Geometry check sheet. Reference: the model listing, model coordinates, mm. A direction names the side the tool comes from. Coordinates: 2 decimals unless noted, no trailing zeros. Loops run counter-clockwise (first coordinate to the right, second up) from the corner with the lowest first, then second, coordinate; pieces in that order, holes last.
from build123d import *

# Parameters (mm, degrees)
SKETCH1_W            = 299.7
SKETCH1_H            = 76.075
BOSS_EXTRUDE1_DEPTH  = 3.175
CUT_EXTRUDE4_DEPTH   = 155.634907221
SKETCH3_R            = 6.5
CUT_EXTRUDE5_DEPTH   = 155.634907221
M4_CLEARANCE_HOLE1_D = 4.5
SKETCH12_W           = 144
SKETCH12_H           = 3.175
BOSS_EXTRUDE2_DEPTH  = 6.35
SKETCH13_R           = 14
CUT_EXTRUDE6_DEPTH   = 157.318115653


with BuildPart() as part:
    # Sketch1 → Boss-Extrude1 (new body)
    with BuildSketch(Plane.XY):
        Rectangle(SKETCH1_W, SKETCH1_H)
    extrude(amount=BOSS_EXTRUDE1_DEPTH)

    # Sketch8 → Cut-Extrude4 (cut, through all)
    with BuildSketch(Plane.XY.offset(3.175)):
        with BuildLine():
            Line((121.65, 18.5125), (123.65, 18.5125))
            ThreePointArc((123.65, 18.5125), (127.185533906, 17.048033906), (128.65, 13.5125))
            Line((128.65, 13.5125), (128.65, -27.282435401))
            ThreePointArc((128.65, -27.282435401), (127.185533906, -30.817969307), (123.65, -32.282435401))
            Line((123.65, -32.282435401), (121.65, -32.282435401))
            ThreePointArc((121.65, -32.282435401), (118.114466094, -30.817969307), (116.65, -27.282435401))
            Line((116.65, -27.282435401), (116.65, 13.5125))
            ThreePointArc((116.65, 13.5125), (118.114466094, 17.048033906), (121.65, 18.5125))
        make_face()
        with BuildLine():
            Line((128.65, -38.0375), (128.65, -27.282435401))
            ThreePointArc((128.65, -27.282435401), (127.185533906, -30.817969307), (123.65, -32.282435401))
            Line((123.65, -32.282435401), (121.65, -32.282435401))
            ThreePointArc((121.65, -32.282435401), (118.114466094, -30.817969307), (116.65, -27.282435401))
            Line((116.65, -27.282435401), (116.65, -38.0375))
            Line((116.65, -38.0375), (128.65, -38.0375))
        make_face()
    cut_extrude4 = extrude(amount=-CUT_EXTRUDE4_DEPTH, mode=Mode.SUBTRACT)

    # Mirror3: Cut-Extrude4 across plane
    add(cut_extrude4.mirror(Plane(origin=(0, 0, 0), x_dir=(0, 0, 1), z_dir=(1, 0, 0))), mode=Mode.SUBTRACT)

    # Sketch3 → Cut-Extrude5 (cut, through all)
    with BuildSketch(Plane(origin=(0, 0, 0), x_dir=(-1, 0, 0), z_dir=(0, 0, -1))):
        with Locations((-97.75, -9.7625)):
            Circle(SKETCH3_R)
        with BuildLine():
            Line((-104.25, -38.0375), (-91.25, -38.0375))
            Line((-91.25, -38.0375), (-91.25, -9.7625))
            ThreePointArc((-91.25, -9.7625), (-97.75, -16.2625), (-104.25, -9.7625))
            Line((-104.25, -9.7625), (-104.25, -38.0375))
        make_face()
        with Locations((97.75, -9.7625)):
            Circle(SKETCH3_R)
        with BuildLine():
            Line((91.25, -38.0375), (104.25, -38.0375))
            Line((104.25, -38.0375), (104.25, -9.7625))
            ThreePointArc((104.25, -9.7625), (97.75, -16.2625), (91.25, -9.7625))
            Line((91.25, -9.7625), (91.25, -38.0375))
        make_face()
    extrude(amount=-CUT_EXTRUDE5_DEPTH, mode=Mode.SUBTRACT)

    # M4 Clearance Hole1 (through all)
    with Locations(Plane(origin=(0, 0, 0), x_dir=(-1, 0, 0), z_dir=(0, 0, -1))):
        with Locations((-85.75, -9.7625), (-109.75, -9.7625), (109.75, -9.7625), (85.75, -9.7625)):
            Hole(M4_CLEARANCE_HOLE1_D / 2)

    # Sketch12 → Boss-Extrude2 (add)
    with BuildSketch(Plane.XZ.offset(38.0375)):
        with Locations((0, 1.5875)):
            Rectangle(SKETCH12_W, SKETCH12_H)
    extrude(amount=BOSS_EXTRUDE2_DEPTH)

    # Sketch13 → Cut-Extrude6 (cut, through all)
    with BuildSketch(Plane(origin=(0, 0, 0), x_dir=(-1, 0, 0), z_dir=(0, 0, -1))):
        with Locations((63.008899223, -6.644651545)):
            Circle(SKETCH13_R)
    cut_extrude6 = extrude(amount=-CUT_EXTRUDE6_DEPTH, mode=Mode.SUBTRACT)

    # Mirror4: Cut-Extrude6 across plane
    add(cut_extrude6.mirror(Plane(origin=(0, 0, 0), x_dir=(0, 0, 1), z_dir=(1, 0, 0))), mode=Mode.SUBTRACT)


solid = part.part
1) Access from +Z, -Z, +X, -X, +Y, -Y to the whole of each face (thin tool, end or side, straight path). Record for faces 4 (the cylindrical face through (76.362, -2.439, 1.565)), 5 (the cylindrical face through (-118.076, 17.009, 1.61)).
Data:
face 4: +Z, -Z
face 5: +Z, -Z, -Y
2) Depth check by flat-ended pin: pin 1 (1 mm diameter, centred on x = 113, z = 1, fed in from -Y); pin 2 (1 mm diameter, centred on x = -122.5, z = 1.5, fed in from -Y). Enter the tip coordinate at first touch or a pass-through.
Data:
pin 1: stops at y = -38.04
pin 2: stops at y = 18.51
3) Section check D-D on z = 2.3. Count the separate pieces of the cut face and the enclosed holes in it, and give its area (3 significant figures).
Data:
separate pieces: 1
enclosed holes: 6
area: 20,200 mm2
4) Section check C-C on y = 4. Record the cut outline in (x, z) (3 decimals).
Data:
outline: (-149.85, 0) - (-128.65, 0) - (-128.65, 3.175) - (-149.85, 3.175) - close; (-116.65, 0) - (-72.102, 0) - (-72.102, 3.175) - (-116.65, 3.175) - close; (-53.915, 0) - (53.915, 0) - (53.915, 3.175) - (-53.915, 3.175) - close; (72.102, 0) - (116.65, 0) - (116.65, 3.175) - (72.102, 3.175) - close; (128.65, 0) - (149.85, 0) - (149.85, 3.175) - (128.65, 3.175) - close
5) Section check B-B on y = -16. Record the cut outline in (x, z) (3 decimals).
Data:
outline: (-149.85, 0) - (-128.65, 0) - (-128.65, 3.175) - (-149.85, 3.175) - close; (-116.65, 0) - (-104.25, 0) - (-104.25, 3.175) - (-116.65, 3.175) - close; (-91.25, 0) - (-73.424, 0) - (-73.424, 3.175) - (-91.25, 3.175) - close; (-52.594, 0) - (52.594, 0) - (52.594, 3.175) - (-52.594, 3.175) - close; (73.424, 0) - (91.25, 0) - (91.25, 3.175) - (73.424, 3.175) - close; (104.25, 0) - (116.65, 0) - (116.65, 3.175) - (104.25, 3.175) - close; (128.65, 0) - (149.85, 0) - (149.85, 3.175) - (128.65, 3.175) - close
6) Material ranges on probe 1 along X at (y, z) = (-30, 0.25); probe 2 along Y at (x, z) = (62, 2.4); probe 3 along Y at (x, z) = (109.75, 1.45), recorded low to high.
Data:
probe 1: x = -149.85 to -128.65, -116.65 to -104.25, -91.25 to 91.25, 104.25 to 116.65, 128.65 to 149.85
probe 2: y = -44.39 to -20.61, 7.32 to 38.04
probe 3: y = -38.04 to -12.01, -7.51 to 38.04
7) Mould release check, pull along Y, two halves, no side actions. Record for faces 1 (the cylindrical face through (-76.362, -2.439, 1.565)), 2 (the flat face through (-2, -3, 3.175)), 3 (the cylindrical face through (127.146, 17.087, 1.61)): +Y half, -Y half, draft (parallel to the pull), parting line (faces both ways), or undercut.
Data:
face 1: undercut
face 2: draft
face 3: -Y half
8) Section check A-A on x = 66. Record the cut outline in (y, z) (1 decimal), and give its area (3 significant figures).
Data:
outline: (-44.4, 0) - (-20.3, 0) - (-20.3, 3.2) - (-44.4, 3.2) - close; (7, 0) - (38, 0) - (38, 3.2) - (7, 3.2) - close
area: 175 mm2
